Model file for the job. Use its own axes, mm. Give positions to 0.01 mm unless a question says otherwise; leave off trailing zeros. Order: outer loops, then holes, each group sorted by start corner. A loop starts at its lowest first (then second) coordinate and runs counter-clockwise, first axis right, second up. Notation, with made-up numbers: (-11.5, 85) -> (23.5, 85) arc R30 ccw to (23.5, 107) -> close; hole circle Ø10 at (64.25, 53.25). An arc over 180 degrees is marked (long way). Use CSV: the item, a comma, the result in double quotes. Start each with the question number.
1. Cut at D-D on z = -1.5. Give the number of separate pieces and of enclosed holes in the cut face, then the cut area to 3 significant figures.
2. Cut at C-C on y = -9. List the corners of the cut face in (x, z) (3 decimals), then the cut area to 3 significant figures.
3. Cut at B-B on x = 0. List the corners of the cut face in (y, z) (1 decimal).
4. Wall check: line 1 (Y direction, x = 0, z = 0.5); line 2 (X direction, y = -23, z = -1.5); line 3 (X direction, y = -20, z = 1). Give the ranges that are in metal, low to high. Write a range as from..to.
5. Cut at A-A on y = 0. List the corners of the cut face in (x, z) (1 decimal), then the cut area to 3 significant figures.
6. Pull direction Y, two halves, no side cores. Call faces 1 (the cylindrical face through (19.866, -8.747, -0.044)), 2 (the cylindrical face through (0.1, 30.16, 0.04)), 3 (the cylindrical face through (2.259, -39.767, 0.044)): released by +Y, released by -Y, zero draft, split by the parting line, or undercut.
7. Drop flat-ended pins along their axis: pin 1 (18.5 mm diameter, centred on x = -4.63, y = -26.26, fed in from +Z) (3 decimals); pin 2 (3 mm diameter, centred on x = -3.74, y = -51.65, fed in from -Z); pin 3 (3 mm diameter, centred on y = -22, z = -2, fed in from +X); pin 4 (3 mm diameter, centred on x = -9.5, z = -0.5, fed in from +Y). Give the stop position or say it passes through.
```python
from build123d import *

# Parameters (mm, degrees)
SKETCH1_R               = 2.4892
SKETCH1_R_2             = 14.2875
BOSS_EXTRUDE1_DEPTH     = 3.175
SKETCH48_R              = 2.4892
BOSS_EXTRUDE2_DEPTH     = 3.175
CUT_EXTRUDE1_DEPTH      = 62.473150941
CUT_EXTRUDE1_DEPTH_BACK = 62.473150941
FILLET1_R               = 6.35


with BuildPart() as part:
    # Sketch1 → Boss-Extrude1 (new, symmetric)
    with BuildSketch(Plane.XY):
        with BuildLine():
            ThreePointArc((4.74437725, 25.815079225), (0, 30.1625), (-4.74437725, 25.815079225))
            Line((-4.74437725, 25.815079225), (-5.256916026, 19.956734205))
            ThreePointArc((-5.256916026, 19.956734205), (-18.703926955, 8.721784377), (-18.666825827, -8.800910167))
            Line((-18.666825827, -8.800910167), (-22.825124901, -12.959209241))
            ThreePointArc((-22.825124901, -12.959209241), (-23.105815516, -19.388081277), (-16.725871077, -20.228016897))
            Line((-16.725871077, -20.228016897), (-11.908664854, -16.854972787))
            ThreePointArc((-11.908664854, -16.854972787), (0, -20.6375), (11.908664854, -16.854972787))
            Line((11.908664854, -16.854972787), (16.725871077, -20.228016897))
            ThreePointArc((16.725871077, -20.228016897), (23.105815516, -19.388081277), (22.825124901, -12.959209241))
            Line((22.825124901, -12.959209241), (18.666825827, -8.800910167))
            ThreePointArc((18.666825827, -8.800910167), (18.703926955, 8.721784377), (5.256916026, 19.956734205))
            Line((5.256916026, 19.956734205), (4.74437725, 25.815079225))
        make_face()
        with Locations((0, 25.4)):
            Circle(SKETCH1_R, mode=Mode.SUBTRACT)
        Circle(SKETCH1_R_2, mode=Mode.SUBTRACT)
        with Locations((-19.457528855, -16.326805286)):
            Circle(SKETCH1_R, mode=Mode.SUBTRACT)
        with Locations((19.457528855, -16.326805286)):
            Circle(SKETCH1_R, mode=Mode.SUBTRACT)
    extrude(amount=BOSS_EXTRUDE1_DEPTH, both=True)

    # Sketch48 → Boss-Extrude2 (add, symmetric)
    with BuildSketch(Plane.XY):
        with BuildLine():
            Line((-10.026080704, -39.562360538), (-8.468509885, -52.230199896))
            ThreePointArc((-8.468509885, -52.230199896), (-3.574599444, -56.408575595), (1.014408673, -51.897457398))
            Line((1.014408673, -51.897457398), (1.680248074, -39.151601649))
            ThreePointArc((1.680248074, -39.151601649), (7.424435707, -34.04649077), (9.71079139, -26.709568641))
            ThreePointArc((9.71079139, -26.709568641), (12.397018184, -21.717853667), (18.000475726, -20.860942737))
            ThreePointArc((18.000475726, -20.860942737), (17.339399127, -20.59235715), (16.725871077, -20.228016897))
            Line((16.725871077, -20.228016897), (11.908664854, -16.854972787))
            ThreePointArc((11.908664854, -16.854972787), (9.92035858, -18.09676468), (7.804051349, -19.105056629))
            ThreePointArc((7.804051349, -19.105056629), (5.636733901, -16.241191156), (2.826163363, -14.005193926))
            ThreePointArc((2.826163363, -14.005193926), (-2.481594068, -14.070335715), (-7.446815831, -12.193342045))
            ThreePointArc((-7.446815831, -12.193342045), (-18.919007392, -24.918243731), (-10.026080704, -39.562360538))
        make_face()
        with Locations((-3.741606205, -51.649004712)):
            Circle(SKETCH48_R, mode=Mode.SUBTRACT)
        with BuildLine():
            ThreePointArc((-8.017864397, -19.016315541), (-3.242789938, -18.386223466), (1.028619665, -20.611849695))
            ThreePointArc((1.028619665, -20.611849695), (-6.021827915, -34.14302987), (-8.017864397, -19.016315541))
        make_face(mode=Mode.SUBTRACT)
    extrude(amount=BOSS_EXTRUDE2_DEPTH, both=True)

    # Sketch48_3 → Cut-Extrude1 (cut, two sides: drawn at the far end of the back side and taken through both)
    with BuildSketch(Plane.XY.offset(-CUT_EXTRUDE1_DEPTH_BACK)):
        with BuildLine():
            ThreePointArc((1.028619665, -20.611849695), (-0.935613673, -19.169949492), (-3.242789938, -18.386223466))
            Line((-3.242789938, -18.386223466), (-3.584524765, -20.323818255))
            ThreePointArc((-3.584524765, -20.323818255), (-1.286041697, -20.597390684), (1.028619665, -20.611849695))
        make_face()
        with BuildLine():
            Line((-3.584524765, -20.323818255), (-3.242789938, -18.386223466))
            ThreePointArc((-3.242789938, -18.386223466), (-5.678872071, -18.333377988), (-8.017864397, -19.016315541))
            ThreePointArc((-8.017864397, -19.016315541), (-5.837914816, -19.794573924), (-3.584524765, -20.323818255))
        make_face()
        with BuildLine():
            ThreePointArc((1.028619665, -20.611849695), (-1.286041697, -20.597390684), (-3.584524765, -20.323818255))
            ThreePointArc((-3.584524765, -20.323818255), (-5.837914816, -19.794573924), (-8.017864397, -19.016315541))
            ThreePointArc((-8.017864397, -19.016315541), (-8.928560564, -33.013124419), (3.367691075, -26.264626668))
            ThreePointArc((3.367691075, -26.264626668), (2.759829762, -23.205822058), (1.028619665, -20.611849695))
        make_face()
    extrude(amount=CUT_EXTRUDE1_DEPTH + CUT_EXTRUDE1_DEPTH_BACK, mode=Mode.SUBTRACT)

    # Fillet1
    fillet1_edges = [part.edges().sort_by_distance(p)[0] for p in [
        (18.666825827, -8.800910167, 0),
        (-18.666825827, -8.800910167, 0),
        (-5.256916026, 19.956734205, 0),
        (5.256916026, 19.956734205, 0),
        (-17.914364977, -20.832363131, 0),
        (-10.026080704, -39.562360538, 0),
        (1.680248074, -39.151601649, 0),
    ]]
    fillet(fillet1_edges, radius=FILLET1_R)


solid = part.part
```
Verdict:
1,separate pieces,"1"
1,enclosed holes,"6"
1,area,"1,390 mm^2"
2,outline,"(-19.936, -3.175) -> (-11.097, -3.175) -> (-11.097, 3.175) -> (-19.936, 3.175) -> close; (11.097, -3.175) -> (19.936, -3.175) -> (19.936, 3.175) -> (11.097, 3.175) -> close"
2,area,"112 mm^2"
3,outline,"(-54.6, -3.2) -> (-32.8, -3.2) -> (-32.8, 3.2) -> (-54.6, 3.2) -> close; (-19.7, -3.2) -> (-14.3, -3.2) -> (-14.3, 3.2) -> (-19.7, 3.2) -> close; (14.3, -3.2) -> (22.9, -3.2) -> (22.9, 3.2) -> (14.3, 3.2) -> close; (27.9, -3.2) -> (30.2, -3.2) -> (30.2, 3.2) -> (27.9, 3.2) -> close"
4,line 1,"-54.6..-32.79, -19.74..-14.29, 14.29..22.91, 27.89..30.16"
4,line 2,"-19.61..-11.94, 2.67..11.05"
4,line 3,"-22.49..-9.61, 0.34..22.49"
5,outline,"(-20.6, -3.2) -> (-14.3, -3.2) -> (-14.3, 3.2) -> (-20.6, 3.2) -> close; (14.3, -3.2) -> (20.6, -3.2) -> (20.6, 3.2) -> (14.3, 3.2) -> close"
5,area,"80.6 mm^2"
6,face 1,"undercut"
6,face 2,"released by +Y"
6,face 3,"released by -Y"
7,pin 1,"z = 3.175"
7,pin 2,"through"
7,pin 3,"x = 21.75"
7,pin 4,"y = 19.07"
